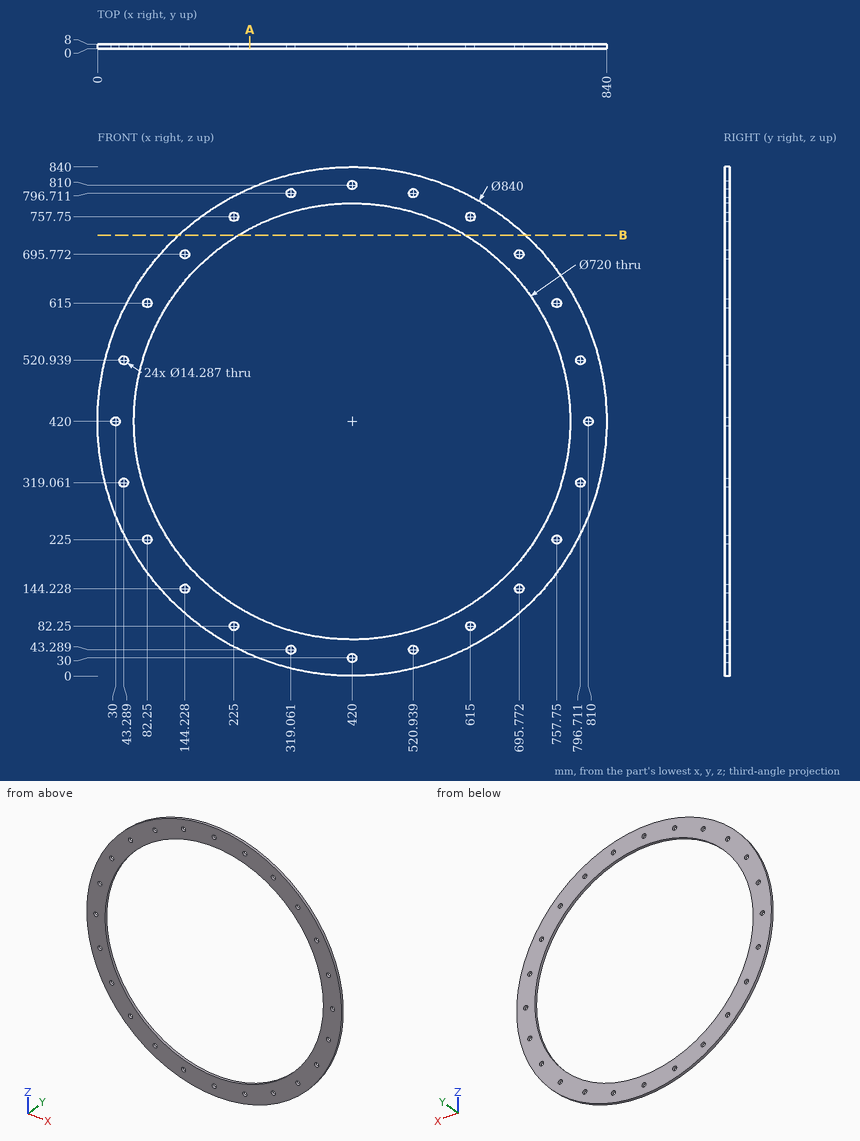
Here's the drawing with two shaded views (mm, measured from the low corner). I have some questions. Round coordinates to 2 decimals unless told otherwise and drop trailing zeros. Loops run counter-clockwise (first coordinate to the right, second up) from the corner with the lowest first, then second, coordinate; pieces in that order, holes last. Notation, with made-up numbers: (-6.5, -40) -> (21.5, -40) arc R11 ccw to (21.5, -24) -> close; hole circle Ø11 at (31, -29.5). An arc over 180 degrees is marked (long way). Answer as CSV lines item,"result". Start each with the question number.
1. I need wall thicknesses on probe 1 along Z at (x, y) = (431, 3.5) (1 decimal); probe 2 along X at (y, z) = (4.75, 692) (1 decimal); probe 3 along X at (y, z) = (1.25, 409.5). Which ranges of each line are inside material? Lowest first, please. Write a range as from..to.
2. I'm going to push flat-ended pins straight in: P1, Ø2, axis at x = 613.5, y = 6.5, coming from the -Z side; P2, Ø3, axis at y = 4.5, z = 382, coming from the -X side; P3, Ø3, axis at x = 112, y = 5, coming from the -Z side (1 decimal). Where does each tip first touch, or does it pass through?
3. Imagine slicing it at B-B on z = 727.5. Write out the boundary of the cut face in (x, y).
4. Imagine slicing it at A-A on x = 251.5. Write out the boundary of the cut face in (y, z).
Solution:
1,probe 1,"0.1..60.2, 779.8..839.9"
1,probe 2,"100..138.2, 150.3..184.2, 655.8..689.7, 701.8..740"
1,probe 3,"0.13..60.15, 779.85..839.87"
2,P1,"z = 46.71"
2,P2,"x = 1.59"
2,P3,"z = 132.8"
3,outline,"(133.92, 0) -> (232.8, 0) -> (232.8, 8) -> (133.92, 8) -> close; (607.2, 0) -> (706.08, 0) -> (706.08, 8) -> (607.2, 8) -> close"
4,outline,"(0, 35.28) -> (8, 35.28) -> (8, 101.87) -> (0, 101.87) -> close; (0, 738.13) -> (8, 738.13) -> (8, 804.72) -> (0, 804.72) -> close"
